```python
from build123d import *

# Parameters (mm, degrees)
F0_R        = 1.6
F0_R_2      = 3
F1_DEPTH    = 4
F2_T1_DEPTH = 4


# Not quite as in the source:
# - a fillet or chamfer that OpenCascade refuses, or shapes differently, is made with other operations: its cross-section is extruded or revolved along the edge and cut away or added


with BuildPart() as f1:
    # F0 (on Top) → F1 (new body)
    with BuildSketch(Plane.XY):
        with BuildLine():
            ThreePointArc((88.7907835501, 77.4770750512), (81.670833227, 81.670833227), (77.4770750512, 88.7907835501))
            Line((77.4770750512, 88.7907835501), (0, 11.313708499))
            Line((0, 11.313708499), (0, 0))
            Line((0, 0), (11.313708499, 0))
            Line((11.313708499, 0), (88.7907835501, 77.4770750512))
        make_face()
        with Locations((4, 4)):
            Circle(F0_R, mode=Mode.SUBTRACT)
        with Locations((15.25, 15.25)):
            Circle(F0_R_2, mode=Mode.SUBTRACT)
        with Locations((26.499998178, 26.499998178)):
            Circle(F0_R, mode=Mode.SUBTRACT)
        with BuildLine():
            ThreePointArc((96.2725882585, 90.4036019747), (90.4036019747, 90.4036019747), (90.4036019747, 96.2725882585))
            Line((90.4036019747, 96.2725882585), (87.6812408671, 98.9949493661))
            Line((87.6812408671, 98.9949493661), (83.6077136088, 94.9214221078))
            ThreePointArc((83.6077136088, 94.9214221078), (83.7226030948, 94.9339214207), (83.8380951166, 94.9380951166))
            Line((83.8380951166, 94.9380951166), (85.3380951166, 94.9380951166))
            ThreePointArc((85.3380951166, 94.9380951166), (86.4694659665, 94.4694659665), (86.9380951166, 93.3380951166))
            ThreePointArc((86.9380951166, 93.3380951166), (86.4694659665, 92.2067242667), (85.3380951166, 91.7380951166))
            Line((85.3380951166, 91.7380951166), (83.8380951166, 91.7380951166))
            ThreePointArc((83.8380951166, 91.7380951166), (82.6280103236, 92.2913407072), (82.2547681255, 93.5684766245))
            Line((82.2547681255, 93.5684766245), (77.4770750512, 88.7907835501))
            ThreePointArc((77.4770750512, 88.7907835501), (81.670833227, 81.670833227), (88.7907835501, 77.4770750512))
            Line((88.7907835501, 77.4770750512), (93.5684766245, 82.2547681255))
            ThreePointArc((93.5684766245, 82.2547681255), (92.2913407072, 82.6280103236), (91.7380951166, 83.8380951166))
            Line((91.7380951166, 83.8380951166), (91.7380951166, 85.3380951166))
            ThreePointArc((91.7380951166, 85.3380951166), (93.3380951166, 86.9380951166), (94.9380951166, 85.3380951166))
            Line((94.9380951166, 85.3380951166), (94.9380951166, 83.8380951166))
            ThreePointArc((94.9380951166, 83.8380951166), (94.9339214207, 83.7226030948), (94.9214221078, 83.6077136088))
            Line((94.9214221078, 83.6077136088), (98.9949493661, 87.6812408671))
            Line((98.9949493661, 87.6812408671), (96.2725882585, 90.4036019747))
        make_face()
        with BuildLine():
            Line((87.6812408671, 98.9949493661), (90.4036019747, 96.2725882585))
            ThreePointArc((90.4036019747, 96.2725882585), (94.9262313609, 97.1721951765), (97.4880951166, 93.3380951166))
            ThreePointArc((97.4880951166, 93.3380951166), (97.1721951765, 91.7499588723), (96.2725882585, 90.4036019747))
            Line((96.2725882585, 90.4036019747), (98.9949493661, 87.6812408671))
            Line((98.9949493661, 87.6812408671), (94.9214221078, 83.6077136088))
            ThreePointArc((94.9214221078, 83.6077136088), (94.4694659665, 82.7067242667), (93.5684766245, 82.2547681255))
            Line((93.5684766245, 82.2547681255), (88.7907835501, 77.4770750512))
            ThreePointArc((88.7907835501, 77.4770750512), (91.5691380282, 76.9331936899), (94.3995707365, 76.8722738645))
            add(Edge.make_bspline(
                [(109.8039163688, 92.2766194967), (99.380066986, 87.2961232472), (94.3995707365, 76.8722738645)],
                knots=[3.9431649716, 3.9431649716, 3.9431649716, 5.4816129892, 5.4816129892, 5.4816129892], degree=2, weights=[1, 0.7184506482, 1]))
            ThreePointArc((109.8039163688, 92.2766194968), (109.829548216, 92.8070822452), (109.8380951166, 93.3380951166))
            ThreePointArc((109.8380951166, 93.3380951166), (104.6238306326, 105.3747962371), (92.2766194968, 109.8039163688))
            add(Edge.make_bspline(
                [(76.8722738645, 94.3995707365), (87.2961232472, 99.380066986), (92.2766194967, 109.8039163688)],
                knots=[0.801572318, 0.801572318, 0.801572318, 2.3400203356, 2.3400203356, 2.3400203356], degree=2, weights=[1, 0.7184506482, 1]))
            ThreePointArc((76.8722738645, 94.3995707365), (76.9331936899, 91.5691380282), (77.4770750512, 88.7907835501))
            Line((77.4770750512, 88.7907835501), (82.2547681255, 93.5684766245))
            ThreePointArc((82.2547681255, 93.5684766245), (82.7067242667, 94.4694659665), (83.6077136088, 94.9214221078))
            Line((83.6077136088, 94.9214221078), (87.6812408671, 98.9949493661))
        make_face()
        with BuildLine():
            ThreePointArc((104.4380951166, 93.3380951166), (103.9694659665, 92.2067242667), (102.8380951166, 91.7380951166))
            Line((102.8380951166, 91.7380951166), (101.3380951166, 91.7380951166))
            ThreePointArc((101.3380951166, 91.7380951166), (99.7380951166, 93.3380951166), (101.3380951166, 94.9380951166))
            Line((101.3380951166, 94.9380951166), (102.8380951166, 94.9380951166))
            ThreePointArc((102.8380951166, 94.9380951166), (103.9694659665, 94.4694659665), (104.4380951166, 93.3380951166))
        make_face(mode=Mode.SUBTRACT)
        with BuildLine():
            Line((91.7380951166, 101.3380951166), (91.7380951166, 102.8380951166))
            ThreePointArc((91.7380951166, 102.8380951166), (93.3380951166, 104.4380951166), (94.9380951166, 102.8380951166))
            Line((94.9380951166, 102.8380951166), (94.9380951166, 101.3380951166))
            ThreePointArc((94.9380951166, 101.3380951166), (93.3380951166, 99.7380951166), (91.7380951166, 101.3380951166))
        make_face(mode=Mode.SUBTRACT)
    extrude(amount=F1_DEPTH)

    # F2: fillet of radius 17.7 on 2 edges, made by hand

    # F2_s2 → F2_t1 (join)
    with BuildSketch(Plane.XY):
        with BuildLine():
            ThreePointArc((83.0395470443, 71.7258385453), (88.2512757036, 75.3327247086), (94.3995707365, 76.8722738645))
            ThreePointArc((94.3995707365, 76.8722738645), (91.5691380282, 76.9331936899), (88.7907835501, 77.4770750512))
            Line((88.7907835501, 77.4770750512), (83.0395470443, 71.7258385453))
        make_face()
        with BuildLine():
            ThreePointArc((76.8722738645, 94.3995707365), (75.3327247086, 88.2512757036), (71.7258385453, 83.0395470443))
            Line((71.7258385453, 83.0395470443), (77.4770750512, 88.7907835501))
            ThreePointArc((77.4770750512, 88.7907835501), (76.9331936899, 91.5691380282), (76.8722738645, 94.3995707365))
        make_face()
    extrude(amount=F2_T1_DEPTH)


solid = f1.part
```
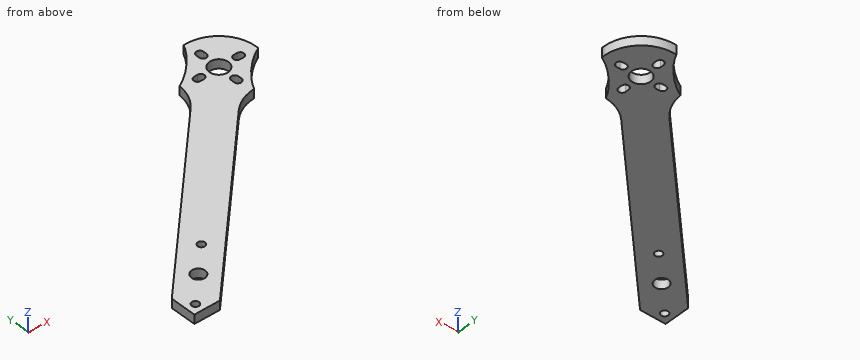
For this review, take the finished solid that the model builds, in its own axes (mm). Round coordinates to 2 decimals unless told otherwise and drop trailing zeros. Write each loop counter-clockwise with the first axis right and the second up, starting at its lowest first coordinate (ties: lowest second). Pieces come first, ordered by that corner, then holes. Notation, with made-up numbers: (-15, 17) -> (16, 17) arc R9 ccw to (16, 23) -> close; hole circle Ø9 at (-9, 0.25). An arc over 180 degrees is marked (long way). Use one line per item in the form item = value.
Q1. Consider section B-B (x = 4). State the section outline as (y, z) points.
Resolved:
outline = (0, 0) -> (2.4, 0) -> (2.4, 4) -> (0, 4) -> close; (5.6, 0) -> (15.31, 0) -> (15.31, 4) -> (5.6, 4) -> close
Q2. Consider section D-D (x = 44). State the section outline as (y, z) points.
Resolved:
outline = (32.69, 0) -> (55.31, 0) -> (55.31, 4) -> (32.69, 4) -> close
Q3. Consider section A-A (y = 15.25). State the section outline as (x, z) points, then the cut area to 3 significant figures.
Resolved:
outline = (3.94, 0) -> (12.25, 0) -> (12.25, 4) -> (3.94, 4) -> close; (18.25, 0) -> (26.56, 0) -> (26.56, 4) -> (18.25, 4) -> close
area = 66.5 mm²
Q4. To check wall thickness, follow probe 1 along X at (y, z) = (12.5, 1.2); probe 2 along Y at (x, z) = (86, 0.45); probe 3 along X at (y, z) = (103, 0.2). State the ranges of each line that lie inside material, in increasing order. Write a range as from..to.
Resolved:
probe_1 = 1.19..14.05, 16.45..23.81
probe_2 = 74.11..91.88, 94.79..101.25
probe_3 = 87.62..91.75, 94.93..106.71
Q5. Consider section C-C (z = 1.2). State how many separate pieces and enclosed holes the cut face has, then the cut area to 3 significant figures.
Resolved:
separate_pieces = 1
enclosed_holes = 8
area = 2,340 mm²
Q6. Clearance check with flat-ended pins moving along their axes: pin 1 Ø1.2 at (x, z) = (102, 1.5) entering from -Y; pin 2 Ø0.8 at (y, z) = (102, 1.5) entering from -X; pin 3 Ø0.8 at (y, z) = (102, 2.5) entering from +X; pin 4 Ø3.5 at (x, y) = (26.5, 26.5) entering from +Z. State where each tip first meets the part, or that it passes through.
Resolved:
pin_1 = 86.14
pin_2 = 86.34
pin_3 = 107.62
pin_4 = 4
